Design review of the part built by this model. Coordinates are the model's own, in mm. A direction names the side the tool comes from. Round coordinates to 2 decimals unless told otherwise and drop trailing zeros. Loops run counter-clockwise (first coordinate to the right, second up) from the corner with the lowest first, then second, coordinate; pieces in that order, holes last. Notation, with made-up numbers: (-24, 13) -> (33, 13) arc R21 ccw to (33, 22) -> close; hole circle Ø9 at (45.5, 5.25). An arc over 180 degrees is marked (long way). Answer as CSV lines item,"result". Start each with the question number.
(1) For P1, Ø0.6, axis at y = -16, z = 0, coming from the +X side; P2, Ø0.6, axis at x = 1.5, y = -18.5, coming from the +Z side; P3, Ø0.6, axis at x = -0.5, y = -11.5, coming from the -Z side, all flat-tipped, find the tip position at first contact; note any pin that passes through.
(2) Take a section at B-B, the plane z = -1.95. Write out the cut boundary in (x, y), and give its area (3 significant figures).
(3) Machinability: for faces 1 (the face through (-0.1, 3.6, 2.5)), 2 (the face through (-2.9, 0.5, -0.1)), which of the approach directions +Z, -Z, +X, -X, +Y, -Y give a long, thin tool a straight path to every point of the face, cutting with its end or side? Answer none if there is none.
(4) Take a section at A-A, the plane y = -13.5. Write out the cut boundary in (x, z), and give its area (3 significant figures).
(5) Take a section at C-C, the plane y = 5. Write out the cut boundary in (x, z).
(6) To check wall thickness, follow line 1 (Z direction, x = 0.2, y = 0.5); line 2 (Z direction, x = -1.7, y = -22.5); line 3 (Y direction, x = -0.55, z = -1.3). State the ranges of each line that lie inside material, in increasing order. Write a range as from..to.
from build123d import *

# Parameters (mm, degrees)
CUT_EXTRUDE1_DEPTH      = 10.618211892
CUT_EXTRUDE1_DEPTH_BACK = 10.618211892
SKETCH3_W               = 0.5
SKETCH3_H               = 0.500000016
BOSS_EXTRUDE2_DEPTH     = 25


with BuildPart() as part:
    # Sketch1 → Revolve1 (revolve)
    with BuildSketch(Plane.XY, mode=Mode.PRIVATE) as revolve1_sk:
        with BuildLine():
            Line((0, 0), (2.9, 0))
            Line((2.9, 0), (2.9, 1))
            Line((2.9, 1), (2.5, 1))
            Line((2.5, 1), (2.5, 6.2))
            ThreePointArc((2.5, 6.2), (1.767766953, 7.967766953), (0, 8.7))
            Line((0, 8.7), (0, 0))
        make_face()
    revolve(revolve1_sk.sketch.rotate(Axis((0, 0, 0), (0, 1, 0)), 90), axis=Axis((0, 0, 0), (0, 1, 0)))

    # Sketch2 → Cut-Extrude1 (cut, two sides: drawn at the far end of the back side and taken through both)
    with BuildSketch(Plane(origin=(0, 0, 0), x_dir=(1, 0, 0), z_dir=(0, 1, 0)).offset(-CUT_EXTRUDE1_DEPTH_BACK)):
        Polygon((2.5, 0), (2.5, 2.5), (3.317010746, 2.5), (3.317010746, -2.186016692), (2.5, -2.186016692), align=None)
    extrude(amount=CUT_EXTRUDE1_DEPTH + CUT_EXTRUDE1_DEPTH_BACK, mode=Mode.SUBTRACT)

    # Sketch3 → Boss-Extrude2 (add)
    with BuildSketch(Plane.XZ):
        with Locations((-1.5, 0)):
            Rectangle(SKETCH3_W, SKETCH3_H)
        with Locations((-0.5, 0)):
            Rectangle(SKETCH3_W, SKETCH3_H)
        with Locations((0.5, 0)):
            Rectangle(SKETCH3_W, SKETCH3_H)
        with Locations((1.5, 0)):
            Rectangle(SKETCH3_W, SKETCH3_H)
    extrude(amount=BOSS_EXTRUDE2_DEPTH)


solid = part.part
The answers:
1,P1,"x = 1.75"
1,P2,"z = 0.25"
1,P3,"z = -0.25"
2,outline,"(-2.15, 0) -> (2.15, 0) -> (2.15, 1) -> (1.56, 1) -> (1.56, 6.2) arc R1.56 ccw to (-1.56, 6.2) -> (-1.56, 1) -> (-2.15, 1) -> close"
2,area,"24.4 mm²"
3,face 1,"+Y"
3,face 2,"+Y, -Y"
4,outline,"(-1.75, -0.25) -> (-1.25, -0.25) -> (-1.25, 0.25) -> (-1.75, 0.25) -> close; (-0.75, -0.25) -> (-0.25, -0.25) -> (-0.25, 0.25) -> (-0.75, 0.25) -> close; (0.25, -0.25) -> (0.75, -0.25) -> (0.75, 0.25) -> (0.25, 0.25) -> close; (1.25, -0.25) -> (1.75, -0.25) -> (1.75, 0.25) -> (1.25, 0.25) -> close"
4,area,"1.00 mm²"
5,outline,"circle Ø5 at (0, 0)"
6,line 1,"-2.89..2.89"
6,line 2,"-0.25..0.25"
6,line 3,"0..8.26"
